Drawing for the job (mm, zero at the part's lowest x, y, z). A direction names the side the tool comes from. Round coordinates to 2 decimals unless told otherwise and drop trailing zeros. Write each loop counter-clockwise with the first axis right and the second up, starting at its lowest first coordinate (ties: lowest second). Pieces come first, ordered by that corner, then holes.
Item 1: Band-saw the part on C-C, the plane z = 7.5. Count the separate pieces of the cut face and the enclosed holes in it, then the cut area to 3 significant figures.
Item 2: Mould opens along Z. For the marked faces 1, 2, 3 and 4 say: +Z half, -Z half, draft (parallel to the pull), parting line (faces both ways), or undercut.
Item 3: Band-saw the part on B-B, the plane y = 1. Write the cut outline in (x, z) (3 decimals), then the cut area to 3 significant figures.
Item 4: Wall check: probe 1 along X at (y, z) = (0.6, 7.5) (3 decimals); probe 2 along X at (y, z) = (4, 7.5); probe 3 along Z at (x, y) = (39, 7.5). Give the ranges that are in metal, low to high.
Item 5: Band-saw the part on D-D, the plane x = 2.5. Write the cut outline in (y, z).
Item 6: Drop flat-ended pins along their axis: pin 1 Ø1.1 at (x, z) = (36.5, 7.5) entering from +Y; pin 2 Ø1.5 at (x, z) = (21.5, 5) entering from +Y; pin 3 Ø2.5 at (x, y) = (40, 6) entering from +Z; pin 4 Ø2 at (y, z) = (6.5, 2.5) entering from +X. Give the stop position or say it passes through.
Item 7: 3-axis set-ups, long thin cutter, end or side, ignore diameter. For the marked faces 5, 6, 7 and 8: which of +Z, -Z, +X, -X, +Y, -Y reach the whole face in a straight line?
Item 8: Band-saw the part on A-A, the plane x = 22. Write the cut outline in (y, z) (3 decimals), then the cut area to 3 significant figures.
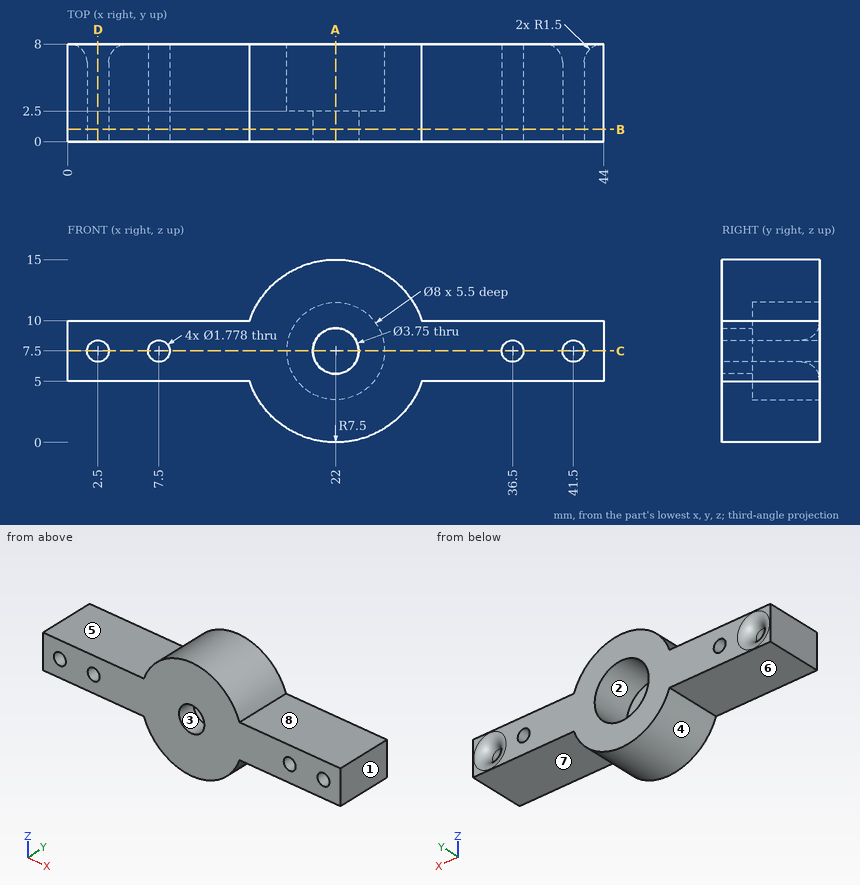
Results:
1. separate pieces: 6
1. enclosed holes: 0
1. area: 240 mm2
2. face 1: draft
2. face 2: undercut
2. face 3: undercut
2. face 4: -Z half
3. outline: (0, 5) - (14.929, 5) arc R7.5 ccw to (29.071, 5) - (44, 5) - (44, 10) - (29.071, 10) arc R7.5 ccw to (14.929, 10) - (0, 10) - close; hole circle Ø1.778 at (2.5, 7.5); hole circle Ø1.778 at (7.5, 7.5); hole circle Ø3.75 at (22, 7.5); hole circle Ø1.778 at (36.5, 7.5); hole circle Ø1.778 at (41.5, 7.5)
3. area: 302 mm2
4. probe 1: x = 0 to 1.611, 3.389 to 6.611, 8.389 to 20.125, 23.875 to 35.611, 37.389 to 40.611, 42.389 to 44
4. probe 2: x = 0 to 1.61, 3.39 to 6.61, 8.39 to 18, 26 to 35.61, 37.39 to 40.61, 42.39 to 44
4. probe 3: z = 5 to 10
5. outline: (0, 5) - (8, 5) - (8, 5.11) arc R1.5 ccw to (6.5, 6.61) - (0, 6.61) - close; (0, 8.39) - (6.5, 8.39) arc R1.5 ccw to (8, 9.89) - (8, 10) - (0, 10) - close
6. pin 1: passes through
6. pin 2: stops at y = 2.5
6. pin 3: stops at z = 10
6. pin 4: stops at x = 28.34
7. face 5: +Z, -X, +Y, -Y
7. face 6: -Z, -X, +Y, -Y
7. face 7: -Z, +X, +Y, -Y
7. face 8: +Z, +X, +Y, -Y
8. outline: (0, 0) - (8, 0) - (8, 3.5) - (2.5, 3.5) - (2.5, 5.625) - (0, 5.625) - close; (0, 9.375) - (2.5, 9.375) - (2.5, 11.5) - (8, 11.5) - (8, 15) - (0, 15) - close
8. area: 66.6 mm2
